```python
from build123d import *

# Parameters (mm, degrees)
CUT_EXTRUDE1_REACH = 51.712
SKETCH2_W          = 22.11
SKETCH2_H          = 3.04
CIRPATTERN1_COUNT  = 4
FILLET1_R          = 1.5


with BuildPart() as part:
    # Sketch1 → Revolve1 (revolve)
    with BuildSketch(Plane.XY):
        with BuildLine():
            Line((0, 24.131243893), (0, 21.131243893))
            Line((0, 21.131243893), (0, 0))
            Line((0, 0), (6, 0))
            Line((6, 0), (6, 21.75))
            ThreePointArc((6, 21.75), (16.839361195, 26.431536124), (24.962781559, 35))
            Line((24.962781559, 35), (21.348078676, 35))
            ThreePointArc((21.348078676, 35), (11.977795315, 27.004824289), (0, 24.131243893))
        make_face()
    revolve(axis=Axis((0, 21.131243893, 0), (0, -1, 0)))

    # Sketch2 → Cut-Extrude1 (cut, up to next)
    with BuildSketch(Plane.XY, mode=Mode.PRIVATE) as cut_extrude1_sk1:
        with Locations((0, 33.48)):
            Rectangle(SKETCH2_W, SKETCH2_H)
    cut_extrude1_tool1 = extrude(cut_extrude1_sk1.sketch, amount=-CUT_EXTRUDE1_REACH, mode=Mode.PRIVATE) & part.part
    cut_extrude1 = cut_extrude1_tool1.solids().sort_by_distance((0, 33.48, 0))[0]
    add(cut_extrude1, mode=Mode.SUBTRACT)

    # CirPattern1: Cut-Extrude1 ×4 about axis
    cirpattern1_axis = Axis((0, 0, 0), (0, 1, 0))
    for i in range(1, CIRPATTERN1_COUNT):
        add(cut_extrude1.rotate(cirpattern1_axis, i * 360 / CIRPATTERN1_COUNT), mode=Mode.SUBTRACT)

    # Fillet1
    fillet1_edges = [part.edges().sort_by_distance(p)[0] for p in [
        (-6, 21.75, 0),
    ]]
    fillet(fillet1_edges, radius=FILLET1_R)


solid = part.part
```
Design review of the part built by this model. Coordinates are the model's own, in mm. A direction names the side the tool comes from. Coordinates: 2 decimals unless noted, no trailing zeros. Write each loop counter-clockwise with the first axis right and the second up, starting at its lowest first coordinate (ties: lowest second). Pieces come first, ordered by that corner, then holes.
1) Insertion check: pin 1 (4 mm diameter, centred on x = -5, z = 19, fed in from +Y); pin 2 (1.5 mm diameter, centred on x = -17, y = 33, fed in from +Z); pin 3 (1 mm diameter, centred on y = 13.5, z = 0.5, fed in from +X). Each pin has a flat end and moves straight along its axis. Give the tip position at first contact, or say it passes through.
2) Add section B-B (x = 10). Write out the cut boundary in (y, z).
3) Mouldability with a two-part tool opening along Z and no side actions: class faces 4 (the cylindrical face through (5.54, 10.42, -2.3)), 5 (the flat face through (0, 31.96, 20)), 6 (the flat face through (-20, 31.96, 0)) as +Z half, -Z half, draft (parallel to the pull), parting line (faces both ways), or undercut.
4) Add section D-D (y = 28.5). Write out the cut boundary in (x, z), plus the area to 3 significant figures.
5) To check wall thickness, follow L1, parallel to Z at x = 0, y = 7.5; L2, parallel to Z at x = -1, y = 15. State the ranges of each line that lie inside material, in increasing order.
6) Machinability: for faces 1 (the flat face through (-17, 35, 17)), 2 (the flat face through (19, 33, 11.055)), 3 (the flat face through (-11.055, 33, 19)), which of the approach directions +Z, -Z, +X, -X, +Y, -Y give a long, thin tool a straight path to every point of the face, cutting with its end or side? Answer none if there is none.
7) Add section A-A (y = 6). Write out the cut boundary in (x, z).
8) Add section C-C (z = -14.5). Write out the cut boundary in (x, y), plus the area to 3 significant figures.
Check result:
1. pin 1: stops at y = 31.96
1. pin 2: stops at z = 17.44
1. pin 3: stops at x = 6
2. outline: (31.96, -20.48) - (31.96, -15.88) arc R24.43 cw to (31.96, 15.88) - (31.96, 20.48) arc R27.65 ccw to start
3. face 4: parting line
3. face 5: draft
3. face 6: undercut
4. outline: circle Ø38.94 at (0, 0); hole circle Ø29.09 at (0, 0)
4. area: 526 mm2
5. L1: z = -6 to 6
5. L2: z = -5.92 to 5.92
6. face 1: +Z, -Z, +X, -X, +Y
6. face 2: +X, -X, +Y
6. face 3: +Z, -Z, +Y
7. outline: circle Ø12 at (0, 0)
8. outline: (-20.32, 35) arc R25.58 ccw to (20.32, 35) - (15.67, 35) arc R22.06 cw to (-15.67, 35) - close
8. area: 144 mm2
